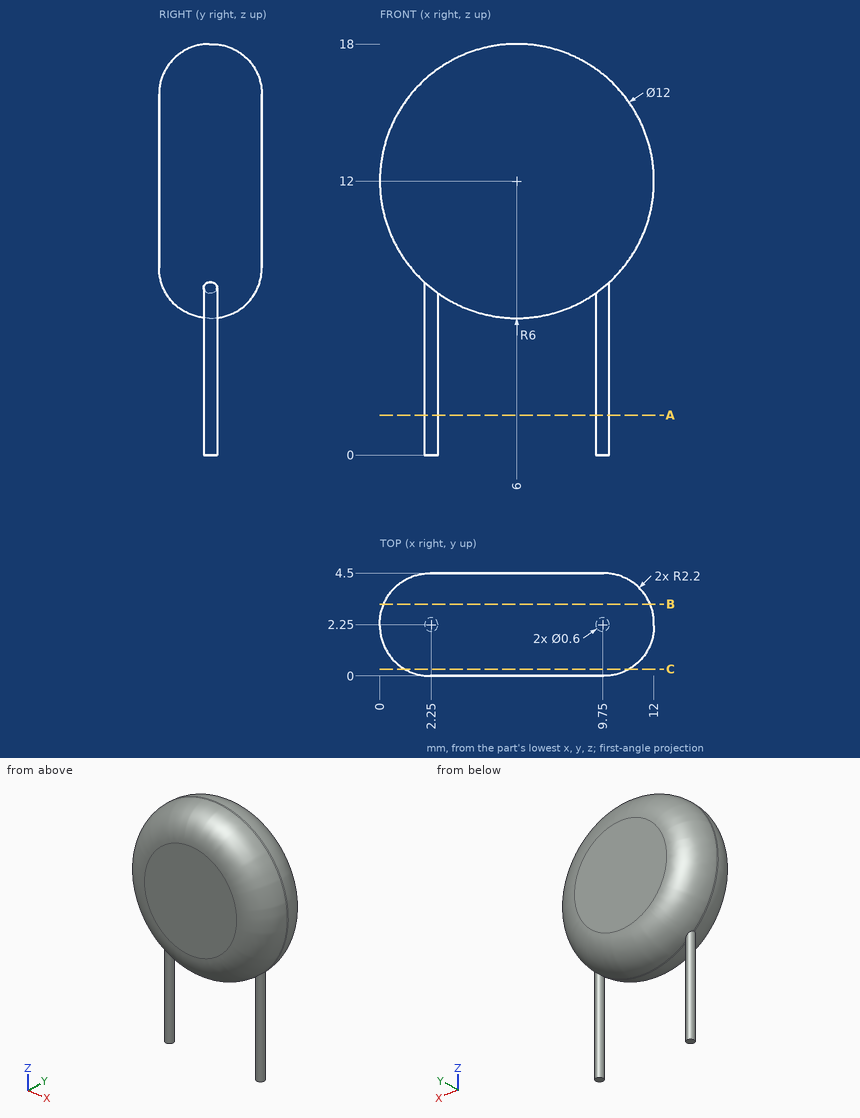
Source: three-view drawing plus pictorial views. Frame: mm from the lowest corner of the part. Coordinates: 2 decimals unless noted, no trailing zeros. Order: outer loops, then holes, each group sorted by start corner. A loop starts at its lowest first (then second) coordinate and runs counter-clockwise, first axis right, second up.
Item 1: Cut plane B-B (y = 3.15). Return loops of the section in (x, z), plus the area to 3 significant figures.
Output values:
outline: circle Ø11.66 at (6, 12)
area: 107 mm2
Item 2: Cut plane C-C (y = 0.3). Return loops of the section in (x, z).
Output values:
outline: circle Ø9.82 at (6, 12)
Item 3: First-contact query: P1, Ø2, axis at x = 9, z = 3.5, coming from the -Y side; P2, Ø1.5, axis at y = 3.5, z = 10, coming from the +X side; P3, Ø2, axis at x = 9.5, z = 16, coming from the -Y side. Flat tips, straight axial feed; report the tip coordinate or a pass-through.
Output values:
P1: stops at y = 1.95
P2: stops at x = 11.71
P3: stops at y = 0.06
Item 4: Material intervals for line 1 (Y direction, x = 5, z = 15.75); line 2 (X direction, y = 2.1, z = 4.5); line 3 (X direction, y = 2.65, z = 13), sorted ascending.
Output values:
line 1: y = 0 to 4.5
line 2: x = 1.99 to 2.51, 9.49 to 10.01
line 3: x = 0.11 to 11.89
Item 5: Cut plane A-A (z = 1.75). Return loops of the section in (x, y).
Output values:
outline: circle Ø0.6 at (2.25, 2.25); circle Ø0.6 at (9.75, 2.25)
